Build history of the part. All positions in model axes, mm. A direction names the side the tool comes from. Round coordinates to 2 decimals unless told otherwise and drop trailing zeros. Write each loop counter-clockwise with the first axis right and the second up, starting at its lowest first coordinate (ties: lowest second). Pieces come first, ordered by that corner, then holes.
from build123d import *

# Parameters (mm, degrees)
SKETCH1_W            = 147.32
SKETCH1_H            = 63.5
BOSS_EXTRUDE3_DEPTH  = 5.08
FILLET4_R            = 12.7
SKETCH4_W            = 121.92
SKETCH4_H            = 63.5
SKETCH4_W_2          = 116.84
SKETCH4_H_2          = 58.42
BOSS_EXTRUDE4_DEPTH  = 30.48
SKETCH9_W            = 10.16
SKETCH9_H            = 10.16
BOSS_EXTRUDE5_DEPTH  = 5.08
FILLET9_R            = 5.08
SKETCH10_R           = 3.175
CUT_EXTRUDE7_DEPTH   = 163.421034352
FILLET12_R           = 7.62
SKETCH11_R           = 3.175
SKETCH11_R_2         = 1.27
BOSS_EXTRUDE7_DEPTH  = 5.08
SKETCH15_R           = 1.27
CUT_EXTRUDE10_DEPTH  = 2.54
BOSS_EXTRUDE9_START  = -2.54
SKETCH16_R           = 3.175
BOSS_EXTRUDE9_DEPTH  = 2.54
SKETCH17_W           = 116.84
SKETCH17_H           = 58.42
CUT_EXTRUDE11_DEPTH  = 5.08
SKETCH18_W           = 116.84
SKETCH18_H           = 58.42
BOSS_EXTRUDE10_DEPTH = 5.08
FILLET16_R           = 5.08
SKETCH13_W           = 7.62
SKETCH13_H           = 10.16
CUT_EXTRUDE12_DEPTH  = 165.316602935
FILLET17_R           = 2.032
CUT_EXTRUDE14_REACH  = 166.317
SKETCH12_W           = 15.24
SKETCH12_H           = 10.16
FILLET18_R           = 2.54


with BuildPart() as part:
    # Sketch1 → Boss-Extrude3 (new body)
    with BuildSketch(Plane(origin=(0, 0, 0), x_dir=(1, 0, 0), z_dir=(0, 1, 0))):
        with Locations((73.66, 31.75)):
            Rectangle(SKETCH1_W, SKETCH1_H)
    extrude(amount=BOSS_EXTRUDE3_DEPTH)

    # Fillet4
    fillet4_edges = [part.edges().sort_by_distance(p)[0] for p in [
        (0, 2.54, -63.5),
        (147.32, 2.54, -63.5),
        (147.32, 2.54, 0),
        (0, 2.54, 0),
    ]]
    fillet(fillet4_edges, radius=FILLET4_R)

    # Sketch4 → Boss-Extrude4 (add)
    with BuildSketch(Plane(origin=(0, 5.08, 0), x_dir=(1, 0, 0), z_dir=(0, 1, 0))):
        with Locations((73.66, 31.75)):
            Rectangle(SKETCH4_W, SKETCH4_H)
        with Locations((73.66, 31.75)):
            Rectangle(SKETCH4_W_2, SKETCH4_H_2, mode=Mode.SUBTRACT)
    extrude(amount=BOSS_EXTRUDE4_DEPTH)

    # Sketch9 → Boss-Extrude5 (add)
    with BuildSketch(Plane(origin=(0, 5.08, 0), x_dir=(1, 0, 0), z_dir=(0, 1, 0))):
        with Locations((20.32, 55.88)):
            Rectangle(SKETCH9_W, SKETCH9_H)
        with Locations((127, 55.88)):
            Rectangle(SKETCH9_W, SKETCH9_H)
        with Locations((127, 7.62)):
            Rectangle(SKETCH9_W, SKETCH9_H)
        with Locations((20.32, 7.62)):
            Rectangle(SKETCH9_W, SKETCH9_H)
    extrude(amount=BOSS_EXTRUDE5_DEPTH)

    # Fillet9
    fillet9_edges = [part.edges().sort_by_distance(p)[0] for p in [
        (25.4, 7.62, -12.7),
        (25.4, 7.62, -50.8),
        (121.92, 7.62, -50.8),
        (121.92, 7.62, -12.7),
    ]]
    fillet(fillet9_edges, radius=FILLET9_R)

    # Sketch10 → Cut-Extrude7 (cut, through all)
    with BuildSketch(Plane(origin=(0, 10.16, 0), x_dir=(1, 0, 0), z_dir=(0, 1, 0))):
        with Locations(Location((20.32, 55.88, 0), (0, 0, 270))):
            Circle(SKETCH10_R)
        with Locations(Location((127, 55.88, 0), (0, 0, 270))):
            Circle(SKETCH10_R)
        with Locations(Location((20.32, 7.62, 0), (0, 0, 270))):
            Circle(SKETCH10_R)
        with Locations(Location((127, 7.62, 0), (0, 0, 270))):
            Circle(SKETCH10_R)
    extrude(amount=-CUT_EXTRUDE7_DEPTH, mode=Mode.SUBTRACT)

    # Fillet12
    fillet12_edges = [part.edges().sort_by_distance(p)[0] for p in [
        (12.7, 20.32, -63.5),
        (12.7, 20.32, 0),
        (134.62, 20.32, 0),
        (134.62, 20.32, -63.5),
    ]]
    fillet(fillet12_edges, radius=FILLET12_R)

    # Sketch11 → Boss-Extrude7 (add)
    # profile 1 of 4: a face of its own
    with BuildSketch(Plane(origin=(0, 10.16, 0), x_dir=(1, 0, 0), z_dir=(0, 1, 0))):
        with Locations(Location((20.32, 55.88, 0), (0, 0, 270))):
            Circle(SKETCH11_R)
        with Locations(Location((20.32, 55.88, 0), (0, 0, 270))):
            Circle(SKETCH11_R_2, mode=Mode.SUBTRACT)
    # profile 2 of 4: a face of its own
    with BuildSketch(Plane(origin=(0, 10.16, 0), x_dir=(1, 0, 0), z_dir=(0, 1, 0))):
        with Locations(Location((127, 55.88, 0), (0, 0, 270))):
            Circle(SKETCH11_R)
        with Locations(Location((127, 55.88, 0), (0, 0, 270))):
            Circle(SKETCH11_R_2, mode=Mode.SUBTRACT)
    # profile 3 of 4: a face of its own
    with BuildSketch(Plane(origin=(0, 10.16, 0), x_dir=(1, 0, 0), z_dir=(0, 1, 0))):
        with Locations(Location((20.32, 7.62, 0), (0, 0, 270))):
            Circle(SKETCH11_R)
        with Locations(Location((20.32, 7.62, 0), (0, 0, 270))):
            Circle(SKETCH11_R_2, mode=Mode.SUBTRACT)
    # profile 4 of 4: a face of its own
    with BuildSketch(Plane(origin=(0, 10.16, 0), x_dir=(1, 0, 0), z_dir=(0, 1, 0))):
        with Locations(Location((127, 7.62, 0), (0, 0, 270))):
            Circle(SKETCH11_R)
        with Locations(Location((127, 7.62, 0), (0, 0, 270))):
            Circle(SKETCH11_R_2, mode=Mode.SUBTRACT)
    extrude(amount=-BOSS_EXTRUDE7_DEPTH)

    # Sketch15 → Cut-Extrude10 (cut)
    with BuildSketch(Plane(origin=(0, 5.08, 0), x_dir=(1, 0, 0), z_dir=(0, 1, 0))):
        with Locations(Location((6.35, 50.8, 0), (0, 0, 270))):
            Circle(SKETCH15_R)
        with Locations(Location((6.35, 12.7, 0), (0, 0, 270))):
            Circle(SKETCH15_R)
        with Locations(Location((140.97, 12.7, 0), (0, 0, 90))):
            Circle(SKETCH15_R)
        with Locations(Location((140.97, 50.8, 0), (0, 0, 90))):
            Circle(SKETCH15_R)
    extrude(amount=-CUT_EXTRUDE10_DEPTH, mode=Mode.SUBTRACT)

    # Sketch16 → Boss-Extrude9 (add)
    with BuildSketch(Plane.XZ.offset(BOSS_EXTRUDE9_START)):
        with Locations(Location((20.32, -7.62, 0), (0, 0, 90))):
            Circle(SKETCH16_R)
        with Locations(Location((127, -7.62, 0), (0, 0, 90))):
            Circle(SKETCH16_R)
        with Locations(Location((20.32, -55.88, 0), (0, 0, 90))):
            Circle(SKETCH16_R)
        with Locations(Location((127, -55.88, 0), (0, 0, 90))):
            Circle(SKETCH16_R)
    extrude(amount=BOSS_EXTRUDE9_DEPTH)

    # Sketch17 → Cut-Extrude11 (cut)
    with BuildSketch(Plane(origin=(0, 10.16, 0), x_dir=(1, 0, 0), z_dir=(0, 1, 0))):
        with Locations((73.66, 31.75)):
            Rectangle(SKETCH17_W, SKETCH17_H)
    extrude(amount=-CUT_EXTRUDE11_DEPTH, mode=Mode.SUBTRACT)

    # Sketch18 → Boss-Extrude10 (add)
    with BuildSketch(Plane(origin=(0, 5.08, 0), x_dir=(1, 0, 0), z_dir=(0, 1, 0))):
        with Locations((73.66, 31.75)):
            Rectangle(SKETCH18_W, SKETCH18_H)
    extrude(amount=-BOSS_EXTRUDE10_DEPTH)

    # Fillet16
    fillet16_edges = [part.edges().sort_by_distance(p)[0] for p in [
        (15.24, 20.32, -2.54),
        (132.08, 20.32, -2.54),
        (132.08, 20.32, -60.96),
        (15.24, 20.32, -60.96),
    ]]
    fillet(fillet16_edges, radius=FILLET16_R)

    # Sketch13 → Cut-Extrude12 (cut, through all)
    with BuildSketch(Plane.XY):
        with Locations((27.94, 15.24)):
            Rectangle(SKETCH13_W, SKETCH13_H)
        with Locations((50.8, 15.24)):
            Rectangle(SKETCH13_W, SKETCH13_H)
    extrude(amount=-CUT_EXTRUDE12_DEPTH, mode=Mode.SUBTRACT)

    # Fillet17
    fillet17_edges = [part.edges().sort_by_distance(p)[0] for p in [
        (24.13, 10.16, -1.27),
        (24.13, 20.32, -1.27),
        (31.75, 20.32, -1.27),
        (31.75, 10.16, -1.27),
        (24.13, 10.16, -62.23),
        (24.13, 20.32, -62.23),
        (31.75, 20.32, -62.23),
        (31.75, 10.16, -62.23),
        (46.99, 10.16, -1.27),
        (46.99, 20.32, -1.27),
        (54.61, 20.32, -1.27),
        (54.61, 10.16, -1.27),
        (46.99, 10.16, -62.23),
        (46.99, 20.32, -62.23),
        (54.61, 20.32, -62.23),
        (54.61, 10.16, -62.23),
    ]]
    fillet(fillet17_edges, radius=FILLET17_R)

    # Sketch12 → Cut-Extrude14 (cut, up to next)
    with BuildSketch(Plane.XY, mode=Mode.PRIVATE) as cut_extrude14_sk1:
        with Locations((107.95, 24.257)):
            Rectangle(SKETCH12_W, SKETCH12_H)
    cut_extrude14_tool1 = extrude(cut_extrude14_sk1.sketch, amount=-CUT_EXTRUDE14_REACH, mode=Mode.PRIVATE) & part.part
    add(cut_extrude14_tool1.solids().sort_by_distance((107.95, 24.257, 0))[0], mode=Mode.SUBTRACT)

    # Fillet18
    fillet18_edges = [part.edges().sort_by_distance(p)[0] for p in [
        (100.33, 19.177, -1.27),
        (100.33, 29.337, -1.27),
        (115.57, 29.337, -1.27),
        (115.57, 19.177, -1.27),
    ]]
    fillet(fillet18_edges, radius=FILLET18_R)


solid = part.part
1) Slice it at B-B (z = -46). Write the cut outline in (x, y), plus the area to 3 significant figures.
Results:
outline: (0, 0) - (147.32, 0) - (147.32, 5.08) - (134.62, 5.08) - (134.62, 35.56) - (132.08, 35.56) - (132.08, 5.08) - (15.24, 5.08) - (15.24, 35.56) - (12.7, 35.56) - (12.7, 5.08) - (0, 5.08) - close
area: 903 mm2
2) Mould opens along Y. For faces 1 (the flat face through (108, 29.337, -1)), 2 (the cylindrical face through (139.899, 3.828, -13.383)), 3 (the flat face through (73, 0, -32)), 4 (the flat face through (28, 20.32, -1)) say: released by +Y, released by -Y, zero draft, split by the parting line, or undercut.
Results:
face 1: undercut
face 2: zero draft
face 3: released by -Y
face 4: undercut
3) Pin check, flat tips, straight feed: pin 1 Ø6 at (y, z) = (30.5, -51.5) entering from -X; pin 2 Ø9 at (y, z) = (27, -33) entering from +X; pin 3 Ø1.3 at (x, z) = (28, -2) entering from -Y; pin 4 Ø10 at (x, z) = (72.5, -35) entering from +Y. Stop position of each tip, or through.
Results:
pin 1: stops at x = 12.7
pin 2: stops at x = 134.62
pin 3: stops at y = 0
pin 4: stops at y = 5.08
4) Which spindle directions (+Z, -Z, +X, -X, +Y, -Y) get a long thin tool onto all of the face, cutting with end or side? Do faces 5 (the flat face through (141, 2.54, -13)), 6 (the flat face through (108, 19.177, -1)), 7 (the flat face through (51, 20.32, -1)). Say none if no direction does.
Results:
face 5: +Y
face 6: +Z
face 7: +Z, -Z
5) Slice it at C-C (x = 79.5). Write the cut outline in (y, z), plus the area to 3 significant figures.
Results:
outline: (0, -63.5) - (35.56, -63.5) - (35.56, -60.96) - (5.08, -60.96) - (5.08, -2.54) - (35.56, -2.54) - (35.56, 0) - (0, 0) - close
area: 477 mm2
6) Wall check: L1, parallel to X at y = 3.4, z = -50.8; L2, parallel to Z at x = 34.5, y = 32; L3, parallel to X at y = 19.5, z = -56. Give the ranges that are in metal, low to high.
Results:
L1: x = 0 to 5.08, 7.62 to 139.7, 142.24 to 147.32
L2: z = -63.5 to -60.96, -2.54 to 0
L3: x = 12.7 to 15.24, 132.08 to 134.62
7) Slice it at A-A (y = 32). Write the cut outline in (x, z).
Results:
outline: (12.7, -55.88) arc R7.62 ccw to (20.32, -63.5) - (127, -63.5) arc R7.62 ccw to (134.62, -55.88) - (134.62, -7.62) arc R7.62 ccw to (127, 0) - (20.32, 0) arc R7.62 ccw to (12.7, -7.62) - close; hole (15.24, -55.88) arc R5.08 ccw to (20.32, -60.96) - (127, -60.96) arc R5.08 ccw to (132.08, -55.88) - (132.08, -7.62) arc R5.08 ccw to (127, -2.54) - (20.32, -2.54) arc R5.08 ccw to (15.24, -7.62) - close
